The drawing under review shows one solid part. Ordinate dimensions are in mm from its lowest x, y, z. Coordinates: 2 decimals unless noted, no trailing zeros. Loops run counter-clockwise (first coordinate to the right, second up) from the corner with the lowest first, then second, coordinate; pieces in that order, holes last. Notation, with made-up numbers: M 84,-16.75 L 112,-16.75 A24 ccw 112,3.25 Z; hole C 52,16 d10. An arc over 180 degrees is marked long. Use one line per item in the form item = value.
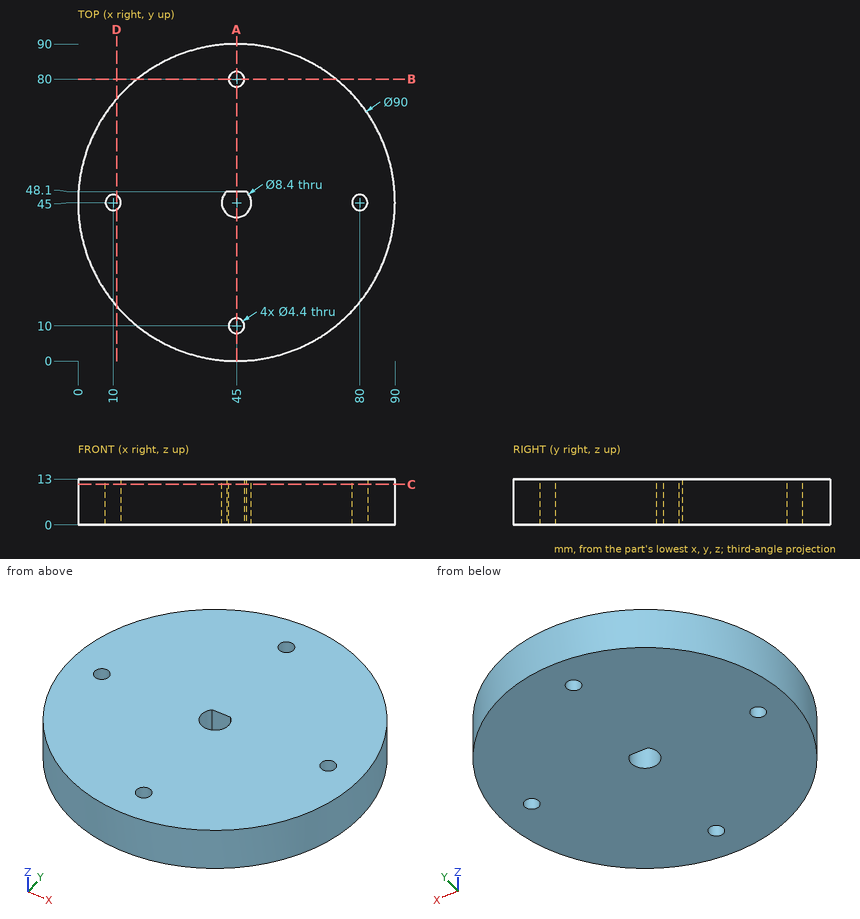
1. For pin 1 Ø3 at (y, z) = (56.5, 3) entering from +X; pin 2 Ø3 at (x, z) = (45.5, 7) entering from -Y; pin 3 Ø5 at (x, y) = (45, 45) entering from -Z; pin 4 Ø5 at (y, z) = (31.5, 1.5) entering from -X, all flat-tipped, find the tip position at first contact; note any pin that passes through.
Computed values:
pin_1 = 88.87
pin_2 = 0
pin_3 = through
pin_4 = 1.37
2. Wall thickness on line 1 along Y through (x, z) = (45, 10); line 2 along X through (y, z) = (78.5, 1.5); line 3 along X through (y, z) = (80, 3.25): over which ranges is each line inside the solid? List them lowest first. Write a range as from..to.
Computed values:
line_1 = 0..7.8, 12.2..40.8, 48.1..77.8, 82.2..90
line_2 = 14.95..43.39, 46.61..75.05
line_3 = 16.72..42.8, 47.2..73.28
3. Consider section C-C on z = 11.5. Write out the cut boundary in (x, y).
Computed values:
outline = C 45,45 d90; hole C 10,45 d4.4; hole M 42.17,48.1 A4.2 ccw long 47.83,48.1 Z; hole C 45,10 d4.4; hole C 45,80 d4.4; hole C 80,45 d4.4
4. Consider section B-B on y = 80. Write out the cut boundary in (x, z), plus the area to 3 significant figures.
Computed values:
outline = M 16.72,0 L 42.8,0 L 42.8,13 L 16.72,13 Z; M 47.2,0 L 73.28,0 L 73.28,13 L 47.2,13 Z
area = 678 mm2
5. Consider section A-A on x = 45. Write out the cut boundary in (y, z), plus the area to 3 significant figures.
Computed values:
outline = M 0,0 L 7.8,0 L 7.8,13 L 0,13 Z; M 12.2,0 L 40.8,0 L 40.8,13 L 12.2,13 Z; M 48.1,0 L 77.8,0 L 77.8,13 L 48.1,13 Z; M 82.2,0 L 90,0 L 90,13 L 82.2,13 Z
area = 961 mm2
6. Consider section D-D on x = 11. Write out the cut boundary in (y, z), plus the area to 4 significant figures.
Computed values:
outline = M 15.52,0 L 43.04,0 L 43.04,13 L 15.52,13 Z; M 46.96,0 L 74.48,0 L 74.48,13 L 46.96,13 Z
area = 715.5 mm2
